Input: dimensioned drawing with shaded views. Units: mm. Origin: part minimum x, y, z. Round coordinates to 2 decimals unless told otherwise and drop trailing zeros. Write each loop counter-clockwise with the first axis right and the second up, starting at its lowest first coordinate (ties: lowest second). Pieces come first, ordered by that corner, then holes. Notation, with made-up numbers: M 27.5,49.5 L 46.5,49.5 A37 cw 46.5,85.5 Z; hole C 12.25,-32 d9. An arc over 180 degrees is marked long. Use one line per item in the form item = value. Start each with the question number.
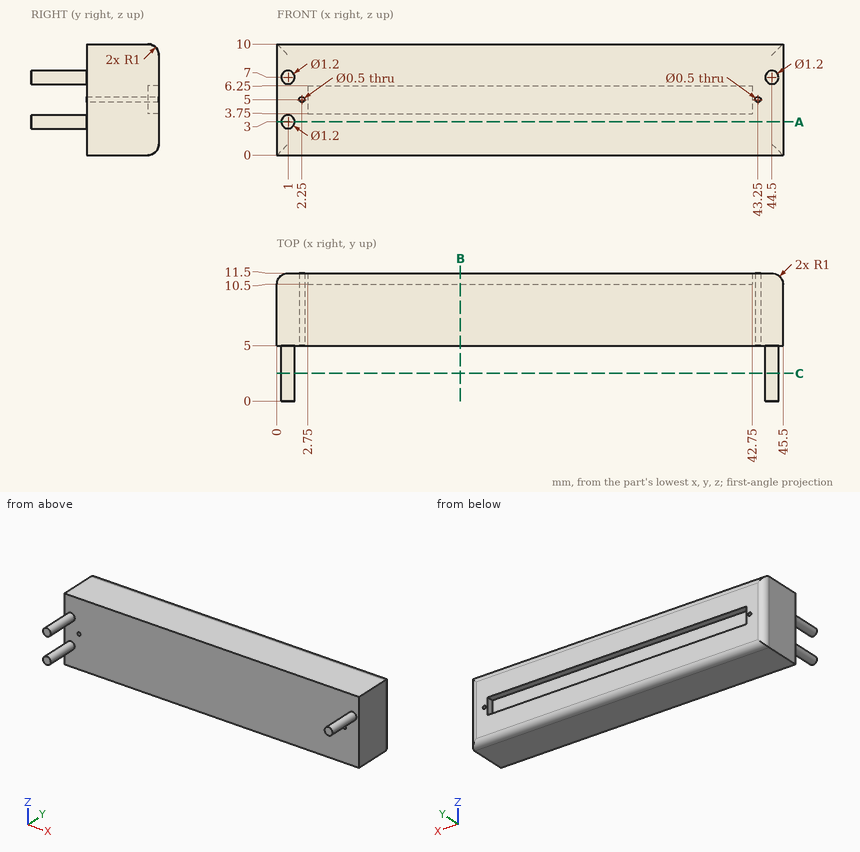
1. Contact query for flat-ended pins moving along their axis: pin 1 (0.8 mm diameter, centred on y = 11, z = 5, fed in from +X) (3 decimals); pin 2 (0.8 mm diameter, centred on x = 16.5, y = 11, fed in from +Z) (3 decimals); pin 3 (3 mm diameter, centred on x = 21, z = 4, fed in from -Y). Output: stop coordinate, or through.
2. Section query A-A (z = 3). Return loops of the section in (x, y).
3. Section query C-C (y = 2.5). Return loops of the section in (x, z), then the cut area to 3 significant figures.
4. Ray query, probe 1 along X at (y, z) = (9.25, 5); probe 2 along Y at (x, z) = (21, 2.25); probe 3 along Z at (x, y) = (43.25, 6.75). Return the intervals inside material, ascending.
5. Section query B-B (x = 16.5). Return loops of the section in (y, z), then the cut area to 3 significant figures.
Checks:
q1.pin_1 = 45.495
q1.pin_2 = 9.995
q1.pin_3 = 5
q2.outline = M 0,5 L 0.4,5 L 0.4,0 L 1.6,0 L 1.6,5 L 45.5,5 L 45.5,10.5 A1 ccw 44.5,11.5 L 1,11.5 A1 ccw 0,10.5 Z
q3.outline = C 1,3 d1.2; C 1,7 d1.2; C 44.5,7 d1.2
q3.area = 3.39 mm^2
q4.probe_1 = 0 to 2, 2.5 to 43, 43.5 to 45.5
q4.probe_2 = 5 to 11.5
q4.probe_3 = 0 to 4.75, 5.25 to 10
q5.outline = M 5,0 L 10.5,0 A1 ccw 11.5,1 L 11.5,3.75 L 10.5,3.75 L 10.5,6.25 L 11.5,6.25 L 11.5,9 A1 ccw 10.5,10 L 5,10 Z
q5.area = 62.1 mm^2
